Read the model definition and answer for the solid it produces. Units are mm, in the model's axes. A direction names the side the tool comes from. Give positions to 0.01 mm unless a question says otherwise; leave off trailing zeros. Loops run counter-clockwise (first coordinate to the right, second up) from the corner with the lowest first, then second, coordinate; pieces in that order, holes last. Notation, with made-up numbers: (52.25, -36) - (69.25, -36) arc R24 ccw to (69.25, -6) - close; hole circle Ø8 at (52, -19.5). An arc over 180 degrees is marked (long way). Put each result on its own line as item: value. Start each with the question number.
1. For faces 5 (the flat face through (0, 3, -2.5)), 6 (the flat face through (0, 20, 0)), determine the directions among +Z, -Z, +X, -X, +Y, -Y from which every point of the face is accessible in a straight line to the end or side of a thin tool.
2. A cutting plane is placed at A-A, the plane y = 5.75. Determine the outline of the cut face in (x, z), plus the area to 3 significant figures.
3. Consider L1, parallel to Z at x = -2.75, y = 4.75; L2, parallel to X at y = 13.25, z = -4; L3, parallel to Z at x = 0.5, y = 1.75. Determine where each line is inside the solid, lowest interval first. Write a range as from..to.
4. A cutting plane is placed at B-B, the plane y = 17.75. Determine the outline of the cut face in (x, z), plus the area to 3 significant figures.
5. For a pull along X with two mould halves and no side action, classify faces 1 (the cylindrical face through (3.233, 17.472, 1.341)), 2 (the flat face through (-1.328, 6, 2.295)), 3 (the flat face through (0, 3, 2.5)), 4 (the flat face through (2, 0, 2)) as released by +X, released by -X, zero draft, split by the parting line, or undercut.
6. Given pin 1 Ø1 at (x, y) = (-2, 2) entering from +Z; pin 2 Ø1.5 at (x, y) = (-1.5, 3) entering from -Z; pin 3 Ø0.6 at (x, z) = (-2.5, 0) entering from -Y, each flat-ended and moving along its own axis, determine where each tip first touches the part or whether it passes through.
7. A cutting plane is placed at C-C, the plane y = 14.5. Determine the outline of the cut face in (x, z), plus the area to 3 significant figures.
```python
from build123d import *

# Parameters (mm, degrees)
SKETCH1_R                 = 5
BOSS_EXTRUDE1_DEPTH       = 15
SKETCH2_R                 = 3.5
BOSS_EXTRUDE2_DEPTH       = 5
FILLET1_R                 = 0.5
F_5_0MM_DOWEL_HOLE2_D     = 5
F_5_0MM_DOWEL_HOLE2_DEPTH = 6
F_5_0MM_DOWEL_HOLE2_TIP   = 1.502151548
CUT_EXTRUDE1_DEPTH        = 6
CHAMFER1_SIZE             = 0.5


with BuildPart() as part:
    # Sketch1 → Boss-Extrude1 (new body)
    with BuildSketch(Plane(origin=(0, 0, 0), x_dir=(1, 0, 0), z_dir=(0, 1, 0))):
        Circle(SKETCH1_R)
    extrude(amount=BOSS_EXTRUDE1_DEPTH)

    # Sketch2 → Boss-Extrude2 (add)
    with BuildSketch(Plane(origin=(0, 15, 0), x_dir=(1, 0, 0), z_dir=(0, 1, 0))):
        Circle(SKETCH2_R)
    extrude(amount=BOSS_EXTRUDE2_DEPTH)

    # Fillet1
    fillet1_edges = [part.edges().sort_by_distance(p)[0] for p in [
        (-3.5, 15, 0),
        (-3.5, 20, 0),
    ]]
    fillet(fillet1_edges, radius=FILLET1_R)

    # Sketch3 → Cut-Revolve1 (revolve, cut)
    with BuildSketch(Plane.XY):
        Polygon((-5, 13.792893219), (-3.646446609, 15.146446609), (-5, 15), align=None)
    revolve(axis=Axis((0, 20, 0), (0, -1, 0)), mode=Mode.SUBTRACT)

    # Ø5.0mm Dowel Hole2
    with Locations(Plane(origin=(0, 0, 0), x_dir=(-1, 0, 0), z_dir=(0, -1, 0))):
        with Locations((0, 0)):
            Hole(F_5_0MM_DOWEL_HOLE2_D / 2, depth=F_5_0MM_DOWEL_HOLE2_DEPTH)
            with Locations((0, 0, -(F_5_0MM_DOWEL_HOLE2_DEPTH + F_5_0MM_DOWEL_HOLE2_TIP / 2))):  # 118° drill point
                Cone(0, F_5_0MM_DOWEL_HOLE2_D / 2, F_5_0MM_DOWEL_HOLE2_TIP, mode=Mode.SUBTRACT)

    # Sketch4 → Cut-Extrude1 (cut)
    with BuildSketch(Plane.XZ):
        Polygon((2.886751346, 0), (1.443375673, 2.5), (-1.443375673, 2.5), (-2.886751346, 0), (-1.443375673, -2.5), (1.443375673, -2.5), align=None)
    extrude(amount=-CUT_EXTRUDE1_DEPTH, mode=Mode.SUBTRACT)

    # Chamfer1
    chamfer1_edges = [part.edges().sort_by_distance(p)[0] for p in [
        (-5, 0, 0),
    ]]
    chamfer(chamfer1_edges, length=CHAMFER1_SIZE)


solid = part.part
```
Return value:
1. face 5: -Y
1. face 6: +Z, -Z, +X, -X, +Y
2. outline: circle Ø10 at (0, 0); hole (-2.89, 0) - (-1.44, -2.5) - (1.44, -2.5) - (2.89, 0) - (1.44, 2.5) - (-1.44, 2.5) - close
2. area: 56.9 mm2
3. L1: z = -4.18..-0.24, 0.24..4.18
3. L2: x = -3..3
3. L3: z = -4.97..-2.5, 2.5..4.97
4. outline: circle Ø7 at (0, 0)
4. area: 38.5 mm2
5. face 1: split by the parting line
5. face 2: undercut
5. face 3: undercut
5. face 4: zero draft
6. pin 1: stops at z = 4.77
6. pin 2: stops at z = -4.94
6. pin 3: stops at y = 6
7. outline: circle Ø8.59 at (0, 0)
7. area: 57.9 mm2
